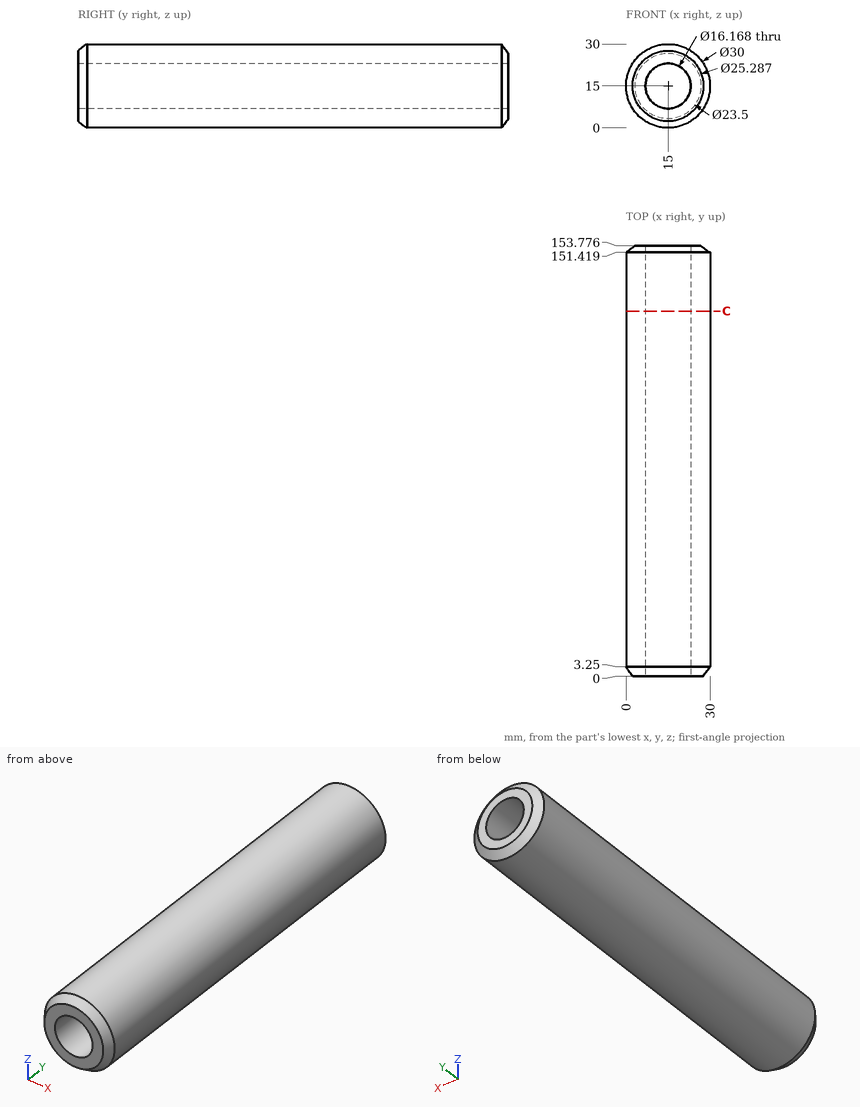
The figure shows three views and two pictorial views of one solid part (mm, origin at its lowest corner). Answer the questions. Coordinates: 2 decimals unless noted, no trailing zeros. Write each loop counter-clockwise with the first axis right and the second up, starting at its lowest first coordinate (ties: lowest second). Pieces come first, ordered by that corner, then holes. Notation, with made-up numbers: (19, -15.5) -> (63, -15.5) arc R26 ccw to (63, 20.5) -> close; hole circle Ø11 at (28.25, 47). An arc over 180 degrees is marked (long way). Answer as a JSON object with one key per item and string values.
Q1. Consider line 1 (X direction, y = 67, z = 15); line 2 (Z direction, x = 13.5, y = 146.5) (1 decimal); line 3 (X direction, y = 138, z = 11) (1 decimal). Determine where each line is inside the solid, lowest interval first. Write a range as [from, to].
The answers:
{"line 1": "x = [0, 6.92], [23.08, 30]", "line 2": "z = [0.1, 7.1], [22.9, 29.9]", "line 3": "x = [0.5, 8], [22, 29.5]"}
Q2. Flat-ended cylindrical pins translate along their axes: pin 1 Ø2 at (y, z) = (108.5, 22) entering from -X; pin 2 Ø4 at (x, z) = (17, 4.5) entering from -Y; pin 3 Ø3 at (x, y) = (4, 83.5) entering from -Z; pin 4 Ø5 at (x, y) = (7, 50.5) entering from +Z (1 decimal). Find the tip coordinate at first contact, or state that the pin passes through.
The answers:
{"pin 1": "stops at x = 1.25", "pin 2": "stops at y = 0", "pin 3": "stops at z = 3.39", "pin 4": "stops at z = 29"}
Q3. The part is cut by section C-C on y = 130.5. Give the vertices of the cut face in (x, z).
The answers:
{"outline": "circle Ø30 at (15, 15); hole circle Ø16.17 at (15, 15)"}
